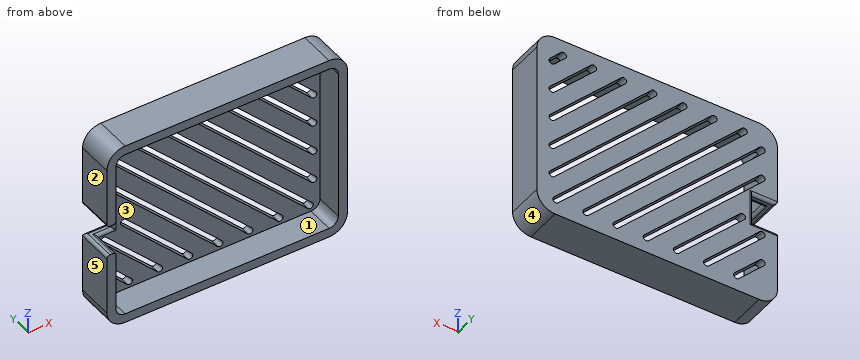
from build123d import *

# Parameters (mm, degrees)
RESSALTO_EXTRUS_O1_DEPTH = 12
CASCA1_T                 = -3
ESBO_O3_W                = 8
ESBO_O3_H                = 10
CORTE_EXTRUS_O2_DEPTH    = 13
FILETE1_R                = 1
CORTE_EXTRUS_O5_REACH    = 14


with BuildPart() as part:
    # Esboço2 → Ressalto-extrusão1 (new body)
    with BuildSketch(Plane(origin=(0, 5.997724004, 0), x_dir=(1, 0, 0), z_dir=(0, 1, 0))):
        with BuildLine():
            Line((-58.558389249, -55.520655269), (-58.558389249, -105.520655269))
            ThreePointArc((-58.558389249, -105.520655269), (-56.801029936, -109.763295956), (-52.558389249, -111.520655269))
            Line((-52.558389249, -111.520655269), (14.441610751, -111.520655269))
            ThreePointArc((14.441610751, -111.520655269), (18.684251438, -109.763295956), (20.441610751, -105.520655269))
            Line((20.441610751, -105.520655269), (20.441610751, -55.520655269))
            ThreePointArc((20.441610751, -55.520655269), (18.684251438, -51.278014582), (14.441610751, -49.520655269))
            Line((14.441610751, -49.520655269), (-52.558389249, -49.520655269))
            ThreePointArc((-52.558389249, -49.520655269), (-56.801029936, -51.278014582), (-58.558389249, -55.520655269))
        make_face()
    extrude(amount=-RESSALTO_EXTRUS_O1_DEPTH)

    # Casca1
    casca1_openings = [part.faces().sort_by_distance(p)[0] for p in [
        (-19.058389249, -6.002275996, 80.520655269),
    ]]
    offset(amount=CASCA1_T, openings=casca1_openings, kind=Kind.INTERSECTION)

    # Esboço3 → Corte-extrusão2 (cut, through all)
    with BuildSketch(Plane(origin=(0, 5.997724004, 0), x_dir=(1, 0, 0), z_dir=(0, 1, 0))):
        with Locations((-54.558389249, -80.520655269)):
            Rectangle(ESBO_O3_W, ESBO_O3_H)
    extrude(amount=-CORTE_EXTRUS_O2_DEPTH, mode=Mode.SUBTRACT)

    # Filete1
    filete1_edges = [part.edges().sort_by_distance(p)[0] for p in [
        (-53.058389249, 2.997724004, 85.520655269),
        (-50.558389249, 2.997724004, 80.520655269),
        (-53.058389249, 2.997724004, 75.520655269),
        (-55.558389249, -1.502275996, 75.520655269),
        (-58.558389249, -0.002275996, 75.520655269),
        (-55.558389249, -1.502275996, 85.520655269),
        (-58.558389249, -0.002275996, 85.520655269),
        (-54.558389249, 5.997724004, 85.520655269),
        (-50.558389249, 5.997724004, 80.520655269),
        (-54.558389249, 5.997724004, 75.520655269),
    ]]
    fillet(filete1_edges, radius=FILETE1_R)

    # Esboço8 → Corte-extrusão5 (cut, up to next)
    with BuildSketch(Plane(origin=(0, 5.997724004, 0), x_dir=(1, 0, 0), z_dir=(0, 1, 0)), mode=Mode.PRIVATE) as corte_extrus_o5_sk1:
        with BuildLine():
            Line((-54.26549603, -62.209172871), (-45.869871648, -53.813548488))
            ThreePointArc((-45.869871648, -53.813548488), (-44.455658085, -53.813548488), (-44.455658085, -55.22776205))
            Line((-44.455658085, -55.22776205), (-52.851282468, -63.623386433))
            ThreePointArc((-52.851282468, -63.623386433), (-54.26549603, -63.623386433), (-54.26549603, -62.209172871))
        make_face()
    corte_extrus_o5_tool1 = extrude(corte_extrus_o5_sk1.sketch, amount=-CORTE_EXTRUS_O5_REACH, mode=Mode.PRIVATE) & part.part
    add(corte_extrus_o5_tool1.solids().sort_by_distance((-49.360577, 5.997724, 58.718467))[0], mode=Mode.SUBTRACT)
    # Esboço8 → Corte-extrusão5 (cut, up to next)
    with BuildSketch(Plane(origin=(0, 5.997724004, 0), x_dir=(1, 0, 0), z_dir=(0, 1, 0)), mode=Mode.PRIVATE) as corte_extrus_o5_sk2:
        with BuildLine():
            Line((-54.26549603, -72.108667807), (-35.970376711, -53.813548488))
            ThreePointArc((-35.970376711, -53.813548488), (-34.556163149, -53.813548488), (-34.556163149, -55.22776205))
            Line((-34.556163149, -55.22776205), (-52.851282468, -73.52288137))
            ThreePointArc((-52.851282468, -73.52288137), (-54.26549603, -73.52288137), (-54.26549603, -72.108667807))
        make_face()
    corte_extrus_o5_tool2 = extrude(corte_extrus_o5_sk2.sketch, amount=-CORTE_EXTRUS_O5_REACH, mode=Mode.PRIVATE) & part.part
    add(corte_extrus_o5_tool2.solids().sort_by_distance((-44.41083, 5.997724, 63.668215))[0], mode=Mode.SUBTRACT)
    # Esboço8 → Corte-extrusão5 (cut, up to next)
    with BuildSketch(Plane(origin=(0, 5.997724004, 0), x_dir=(1, 0, 0), z_dir=(0, 1, 0)), mode=Mode.PRIVATE) as corte_extrus_o5_sk3:
        with BuildLine():
            Line((-47.76549603, -75.508162744), (-26.070881774, -53.813548488))
            ThreePointArc((-26.070881774, -53.813548488), (-24.656668212, -53.813548488), (-24.656668212, -55.22776205))
            Line((-24.656668212, -55.22776205), (-46.351282468, -76.922376306))
            ThreePointArc((-46.351282468, -76.922376306), (-47.76549603, -76.922376306), (-47.76549603, -75.508162744))
        make_face()
    corte_extrus_o5_tool3 = extrude(corte_extrus_o5_sk3.sketch, amount=-CORTE_EXTRUS_O5_REACH, mode=Mode.PRIVATE) & part.part
    add(corte_extrus_o5_tool3.solids().sort_by_distance((-36.211082, 5.997724, 65.367962))[0], mode=Mode.SUBTRACT)
    # Esboço8 → Corte-extrusão5 (cut, up to next)
    with BuildSketch(Plane(origin=(0, 5.997724004, 0), x_dir=(1, 0, 0), z_dir=(0, 1, 0)), mode=Mode.PRIVATE) as corte_extrus_o5_sk4:
        with BuildLine():
            Line((-54.26549603, -91.90765768), (-16.171386838, -53.813548488))
            ThreePointArc((-16.171386838, -53.813548488), (-14.757173275, -53.813548488), (-14.757173275, -55.22776205))
            Line((-14.757173275, -55.22776205), (-52.851282468, -93.321871243))
            ThreePointArc((-52.851282468, -93.321871243), (-54.26549603, -93.321871243), (-54.26549603, -91.90765768))
        make_face()
    corte_extrus_o5_tool4 = extrude(corte_extrus_o5_sk4.sketch, amount=-CORTE_EXTRUS_O5_REACH, mode=Mode.PRIVATE) & part.part
    add(corte_extrus_o5_tool4.solids().sort_by_distance((-34.511335, 5.997724, 73.56771))[0], mode=Mode.SUBTRACT)
    # Esboço8 → Corte-extrusão5 (cut, up to next)
    with BuildSketch(Plane(origin=(0, 5.997724004, 0), x_dir=(1, 0, 0), z_dir=(0, 1, 0)), mode=Mode.PRIVATE) as corte_extrus_o5_sk5:
        with BuildLine():
            Line((-4.857678339, -55.22776205), (-52.851282468, -103.221366179))
            ThreePointArc((-52.851282468, -103.221366179), (-54.26549603, -103.221366179), (-54.26549603, -101.807152617))
            Line((-54.26549603, -101.807152617), (-6.271891901, -53.813548488))
            ThreePointArc((-6.271891901, -53.813548488), (-4.857678339, -53.813548488), (-4.857678339, -55.22776205))
        make_face()
    corte_extrus_o5_tool5 = extrude(corte_extrus_o5_sk5.sketch, amount=-CORTE_EXTRUS_O5_REACH, mode=Mode.PRIVATE) & part.part
    add(corte_extrus_o5_tool5.solids().sort_by_distance((-29.561587, 5.997724, 78.517457))[0], mode=Mode.SUBTRACT)
    # Esboço8 → Corte-extrusão5 (cut, up to next)
    with BuildSketch(Plane(origin=(0, 5.997724004, 0), x_dir=(1, 0, 0), z_dir=(0, 1, 0)), mode=Mode.PRIVATE) as corte_extrus_o5_sk6:
        with BuildLine():
            Line((-48.372396965, -105.813548488), (3.627603035, -53.813548488))
            ThreePointArc((3.627603035, -53.813548488), (5.041816598, -53.813548488), (5.041816598, -55.22776205))
            Line((5.041816598, -55.22776205), (-46.958183402, -107.22776205))
            ThreePointArc((-46.958183402, -107.22776205), (-48.372396965, -107.22776205), (-48.372396965, -105.813548488))
        make_face()
    corte_extrus_o5_tool6 = extrude(corte_extrus_o5_sk6.sketch, amount=-CORTE_EXTRUS_O5_REACH, mode=Mode.PRIVATE) & part.part
    add(corte_extrus_o5_tool6.solids().sort_by_distance((-21.66529, 5.997724, 80.520655))[0], mode=Mode.SUBTRACT)
    # Esboço8 → Corte-extrusão5 (cut, up to next)
    with BuildSketch(Plane(origin=(0, 5.997724004, 0), x_dir=(1, 0, 0), z_dir=(0, 1, 0)), mode=Mode.PRIVATE) as corte_extrus_o5_sk7:
        with BuildLine():
            Line((14.941311534, -55.22776205), (-37.058688466, -107.22776205))
            ThreePointArc((-37.058688466, -107.22776205), (-38.472902028, -107.22776205), (-38.472902028, -105.813548488))
            Line((-38.472902028, -105.813548488), (13.527097972, -53.813548488))
            ThreePointArc((13.527097972, -53.813548488), (14.941311534, -53.813548488), (14.941311534, -55.22776205))
        make_face()
    corte_extrus_o5_tool7 = extrude(corte_extrus_o5_sk7.sketch, amount=-CORTE_EXTRUS_O5_REACH, mode=Mode.PRIVATE) & part.part
    add(corte_extrus_o5_tool7.solids().sort_by_distance((-11.765795, 5.997724, 80.520655))[0], mode=Mode.SUBTRACT)
    # Esboço8 → Corte-extrusão5 (cut, up to next)
    with BuildSketch(Plane(origin=(0, 5.997724004, 0), x_dir=(1, 0, 0), z_dir=(0, 1, 0)), mode=Mode.PRIVATE) as corte_extrus_o5_sk8:
        with BuildLine():
            Line((-28.573407091, -105.813548488), (14.73450397, -62.505637427))
            ThreePointArc((14.73450397, -62.505637427), (16.148717532, -62.505637427), (16.148717532, -63.919850989))
            Line((16.148717532, -63.919850989), (-27.159193529, -107.22776205))
            ThreePointArc((-27.159193529, -107.22776205), (-28.573407091, -107.22776205), (-28.573407091, -105.813548488))
        make_face()
    corte_extrus_o5_tool8 = extrude(corte_extrus_o5_sk8.sketch, amount=-CORTE_EXTRUS_O5_REACH, mode=Mode.PRIVATE) & part.part
    add(corte_extrus_o5_tool8.solids().sort_by_distance((-6.212345, 5.997724, 84.8667))[0], mode=Mode.SUBTRACT)
    # Esboço8 → Corte-extrusão5 (cut, up to next)
    with BuildSketch(Plane(origin=(0, 5.997724004, 0), x_dir=(1, 0, 0), z_dir=(0, 1, 0)), mode=Mode.PRIVATE) as corte_extrus_o5_sk9:
        with BuildLine():
            Line((16.148717532, -73.819345926), (-17.259698592, -107.22776205))
            ThreePointArc((-17.259698592, -107.22776205), (-18.673912155, -107.22776205), (-18.673912155, -105.813548488))
            Line((-18.673912155, -105.813548488), (14.73450397, -72.405132363))
            ThreePointArc((14.73450397, -72.405132363), (16.148717532, -72.405132363), (16.148717532, -73.819345926))
        make_face()
    corte_extrus_o5_tool9 = extrude(corte_extrus_o5_sk9.sketch, amount=-CORTE_EXTRUS_O5_REACH, mode=Mode.PRIVATE) & part.part
    add(corte_extrus_o5_tool9.solids().sort_by_distance((-1.262597, 5.997724, 89.816447))[0], mode=Mode.SUBTRACT)
    # Esboço8 → Corte-extrusão5 (cut, up to next)
    with BuildSketch(Plane(origin=(0, 5.997724004, 0), x_dir=(1, 0, 0), z_dir=(0, 1, 0)), mode=Mode.PRIVATE) as corte_extrus_o5_sk10:
        with BuildLine():
            Line((-8.774417218, -105.813548488), (14.73450397, -82.3046273))
            ThreePointArc((14.73450397, -82.3046273), (16.148717532, -82.3046273), (16.148717532, -83.718840862))
            Line((16.148717532, -83.718840862), (-7.360203656, -107.22776205))
            ThreePointArc((-7.360203656, -107.22776205), (-8.774417218, -107.22776205), (-8.774417218, -105.813548488))
        make_face()
    corte_extrus_o5_tool10 = extrude(corte_extrus_o5_sk10.sketch, amount=-CORTE_EXTRUS_O5_REACH, mode=Mode.PRIVATE) & part.part
    add(corte_extrus_o5_tool10.solids().sort_by_distance((3.68715, 5.997724, 94.766195))[0], mode=Mode.SUBTRACT)
    # Esboço8 → Corte-extrusão5 (cut, up to next)
    with BuildSketch(Plane(origin=(0, 5.997724004, 0), x_dir=(1, 0, 0), z_dir=(0, 1, 0)), mode=Mode.PRIVATE) as corte_extrus_o5_sk11:
        with BuildLine():
            Line((16.148717532, -93.618335799), (2.539291281, -107.22776205))
            ThreePointArc((2.539291281, -107.22776205), (1.125077719, -107.22776205), (1.125077719, -105.813548488))
            Line((1.125077719, -105.813548488), (14.73450397, -92.204122237))
            ThreePointArc((14.73450397, -92.204122237), (16.148717532, -92.204122237), (16.148717532, -93.618335799))
        make_face()
    corte_extrus_o5_tool11 = extrude(corte_extrus_o5_sk11.sketch, amount=-CORTE_EXTRUS_O5_REACH, mode=Mode.PRIVATE) & part.part
    add(corte_extrus_o5_tool11.solids().sort_by_distance((8.636898, 5.997724, 99.715942))[0], mode=Mode.SUBTRACT)
    # Esboço8 → Corte-extrusão5 (cut, up to next)
    with BuildSketch(Plane(origin=(0, 5.997724004, 0), x_dir=(1, 0, 0), z_dir=(0, 1, 0)), mode=Mode.PRIVATE) as corte_extrus_o5_sk12:
        with BuildLine():
            Line((11.024572655, -105.813548488), (14.73450397, -102.103617173))
            ThreePointArc((14.73450397, -102.103617173), (16.148717532, -102.103617173), (16.148717532, -103.517830736))
            Line((16.148717532, -103.517830736), (12.438786218, -107.22776205))
            ThreePointArc((12.438786218, -107.22776205), (11.024572655, -107.22776205), (11.024572655, -105.813548488))
        make_face()
    corte_extrus_o5_tool12 = extrude(corte_extrus_o5_sk12.sketch, amount=-CORTE_EXTRUS_O5_REACH, mode=Mode.PRIVATE) & part.part
    add(corte_extrus_o5_tool12.solids().sort_by_distance((13.586645, 5.997724, 104.66569))[0], mode=Mode.SUBTRACT)


solid = part.part
Geometry check sheet. Reference: the model listing, model coordinates, mm. Face numbers are marked on the shaded views. A direction names the side the tool comes from. Round coordinates to 2 decimals unless told otherwise and drop trailing zeros. Write each loop counter-clockwise with the first axis right and the second up, starting at its lowest first coordinate (ties: lowest second). Pieces come first, ordered by that corner, then holes.
Item 1: Material ranges on line 1 along Z through (x, y) = (-7, -3.5); line 2 along X through (y, z) = (1, 90.5); line 3 along Z through (x, y) = (15.5, 5), recorded low to high.
Determined:
line 1: z = 49.52 to 52.52, 108.52 to 111.52
line 2: x = -58.56 to -55.56, 17.44 to 20.44
line 3: z = 49.61 to 62.21, 64.57 to 72.11, 74.47 to 82.01, 84.37 to 91.91, 94.27 to 101.81, 104.17 to 111.43
Item 2: Access from +Z, -Z, +X, -X, +Y, -Y to the whole of each face (thin tool, end or side, straight path). Record for the marked faces 1 and 2.
Determined:
face 1: -Y
face 2: +Z, -Z, -X, +Y, -Y
Item 3: Mould release check, pull along X, two halves, no side actions. Record for the marked faces 3, 4 and 5: +X half, -X half, draft (parallel to the pull), parting line (faces both ways), or undercut.
Determined:
face 3: undercut
face 4: +X half
face 5: -X half
Item 4: Section check A-A (y = 0.5). Record the boundary of the cut face in (x, z), plus the area to 3 significant figures.
Determined:
outline: (-58.56, 55.52) arc R6 ccw to (-52.56, 49.52) - (14.44, 49.52) arc R6 ccw to (20.44, 55.52) - (20.44, 105.52) arc R6 ccw to (14.44, 111.52) - (-52.56, 111.52) arc R6 ccw to (-58.56, 105.52) - (-58.56, 86.52) arc R1 ccw to (-57.56, 85.52) - (-56.56, 85.52) arc R1 ccw to (-55.56, 86.52) - (-55.56, 105.52) arc R3 cw to (-52.56, 108.52) - (14.44, 108.52) arc R3 cw to (17.44, 105.52) - (17.44, 55.52) arc R3 cw to (14.44, 52.52) - (-52.56, 52.52) arc R3 cw to (-55.56, 55.52) - (-55.56, 74.52) arc R1 ccw to (-56.56, 75.52) - (-57.56, 75.52) arc R1 ccw to (-58.56, 74.52) - close
area: 756 mm2
Item 5: Section check B-B (z = 59.5). Give the number of separate pieces and of enclosed holes in the cut face, plus the area to 3 significant figures.
Determined:
separate pieces: 8
enclosed holes: 0
area: 232 mm2
Item 6: Go/stop test with flat-tipped pins: pin 1 Ø8 at (x, z) = (-18, 66) entering from +Y; pin 2 Ø3 at (x, z) = (-44, 74) entering from -Y; pin 3 Ø0.5 at (y, z) = (4.5, 78.5) entering from -X. Record where each tip stops, or that it passes through.
Determined:
pin 1: stops at y = 6
pin 2: stops at y = 3
pin 3: stops at x = -50.56
